Check sheet for the modelled part. Datum: model origin and axes. Units: mm. Coordinates: 2 decimals unless noted, no trailing zeros. Write each loop counter-clockwise with the first axis right and the second up, starting at its lowest first coordinate (ties: lowest second). Pieces come first, ordered by that corner, then holes. Notation, with made-up numbers: (24.25, 53.5) - (63.25, 53.5) arc R9 cw to (63.25, 70.5) - close; hole circle Ø8 at (24.5, 17.25). An arc over 180 degrees is marked (long way). Use one line per item in the form item = value. Start each with the question number.
1. Draft check along Y on faces 1 (the face through (-1.15, -0.88, 0.24)), 2 (the face through (-2.301, -1.764, 0.244)), 3 (the face through (2, 0, -0.475)). Enter one of: +Y half, -Y half, draft (parallel to the pull), parting line (faces both ways), or undercut.
2. Cross-section at A-A on y = 0. Record the boundary of the cut face in (x, z).
3. Cross-section at C-C on z = 0.4. Record the boundary of the cut face in (x, y), then the cut area to 3 significant figures.
4. Scan lines: line 1 along Y through (x, z) = (0, 0.6); line 2 along X through (y, z) = (0.6, 0.4); line 3 along X through (y, z) = (-0.85, 0.5). Record each from-to range of solid material in increasing order.
```python
from build123d import *

# Parameters (mm, degrees)
SKETCH1_R           = 1
SKETCH1_R_2         = 0.5
BOSS_EXTRUDE1_DEPTH = 0.5
CHAMFER1_SIZE       = 0.1
SCALE1_SCALE        = 1.9329
SCALE2_SCALE        = 1.5


with BuildPart() as part:
    # Sketch1 → Boss-Extrude1 (new body)
    with BuildSketch(Plane.XY):
        Circle(SKETCH1_R)
        Circle(SKETCH1_R_2, mode=Mode.SUBTRACT)
    extrude(amount=BOSS_EXTRUDE1_DEPTH)

    # Chamfer1
    chamfer1_edges = [part.edges().sort_by_distance(p)[0] for p in [
        (-1, 0, 0),
        (-1, 0, 0.5),
    ]]
    chamfer(chamfer1_edges, length=CHAMFER1_SIZE)


with BuildPart() as part_1:
    # Scale1: scaled about (0, 0, 0.25)
    add(part.part.scale(SCALE1_SCALE).moved(Location((0, 0, -0.233225))))


with BuildPart() as part_2:
    # Scale2: scaled about (0, 0, 0.25)
    add(part_1.part.scale(SCALE2_SCALE).moved(Location((0, 0, -0.125))))


solid = part_2.part
```
Final values:
q1.face_1 = undercut
q1.face_2 = parting line
q1.face_3 = draft
q2.outline = (-2.9, -0.18) - (-2.61, -0.47) - (-1.45, -0.47) - (-1.45, 0.97) - (-2.61, 0.97) - (-2.9, 0.68) - close; (1.45, -0.47) - (2.61, -0.47) - (2.9, -0.18) - (2.9, 0.68) - (2.61, 0.97) - (1.45, 0.97) - close
q3.outline = circle Ø5.8 at (0, 0); hole circle Ø2.9 at (0, 0)
q3.area = 19.8 mm²
q4.line_1 = -2.9 to -1.45, 1.45 to 2.9
q4.line_2 = -2.84 to -1.32, 1.32 to 2.84
q4.line_3 = -2.77 to -1.17, 1.17 to 2.77
